from build123d import *

# Parameters (mm, degrees)
F0_W     = 50.8
F0_H     = 101.6
F1_DEPTH = 63.5
F2_R     = 12.7
F3_DEPTH = 96.52
F4_R     = 2.54
F5_DEPTH = 36.322
F6_R     = 6.35
F7_DEPTH = 12.7
F8_R     = 5.08


with BuildPart() as f1:
    # F0 (on Top) → F1 (new body)
    with BuildSketch(Plane.XY):
        Rectangle(F0_W, F0_H)
    extrude(amount=F1_DEPTH)

    # F2 (on face) → F3 (cut)
    with BuildSketch(Plane.XZ.offset(50.8)):
        with Locations((0, 25.4)):
            Circle(F2_R)
    extrude(amount=-F3_DEPTH, mode=Mode.SUBTRACT)

    # F4 (on face) → F5 (cut)
    with BuildSketch(Plane.XY.offset(63.5)):
        with Locations((0, 40.64)):
            Circle(F4_R)
    extrude(amount=-F5_DEPTH, mode=Mode.SUBTRACT)

    # F6 (on face) → F7 (cut)
    with BuildSketch(Plane.XY.offset(63.5)):
        Circle(F6_R)
    extrude(amount=-F7_DEPTH, mode=Mode.SUBTRACT)

    # F8
    f8_edges = [f1.edges().sort_by_distance(p)[0] for p in [
        (25.4, -50.8, 31.75),
        (-25.4, -50.8, 31.75),
        (-25.4, 50.8, 31.75),
        (-25.4, 0, 0),
        (0, 50.8, 0),
        (25.4, 50.8, 31.75),
        (25.4, 0, 0),
        (0, -50.8, 0),
    ]]
    fillet(f8_edges, radius=F8_R)


solid = f1.part
Model file for the job. Use its own axes, mm. A direction names the side the tool comes from. Round coordinates to 2 decimals unless told otherwise and drop trailing zeros. Order: outer loops, then holes, each group sorted by start corner. A loop starts at its lowest first (then second) coordinate and runs counter-clockwise, first axis right, second up.
(1) Band-saw the part on A-A (x = 0). List the corners of the cut face in (y, z).
(2) Drill centre lines: line 1 (X direction, y = 40.64, z = 48.25); line 2 (Y direction, x = 0, z = 49); line 3 (Z direction, x = 0, y = -18). Where is each one in solid material? Low to high.
(3) Pin check, flat tip, straight feed: pin 1 (7.5 mm diameter, centred on x = -2.5, z = 22, fed in from -Y). Stop position of the tip, or through.
(4) 3-axis set-ups, long thin cutter, end or side, ignore diameter. For faces 1 (the face through (5.86, -3.216, 14.133)), 2 (the face through (1.37, 42.78, 50.85)), 3 (the face through (23.872, 0.64, 1.449)): which of +Z, -Z, +X, -X, +Y, -Y reach the whole face in a straight line?
(5) Band-saw the part on B-B (y = 0). List the corners of the cut face in (x, z), then the cut area to 3 significant figures.
(6) Band-saw the part on C-C (z = 25.4). List the corners of the cut face in (x, y).
(7) Pull direction X, two halves, no side cores. Call faces 4 (the face through (-1.38, -6.2, 57.24)), 5 (the face through (0, 50.8, 34)), 6 (the face through (23.872, 49.351, 34.699)): released by +X, released by -X, zero draft, split by the parting line, or undercut.
(8) Band-saw the part on D-D (y = 40.64). List the corners of the cut face in (x, z), then the cut area to 3 significant figures.
Verdict:
1. outline: (-50.8, 5.08) arc R5.08 ccw to (-45.72, 0) - (45.72, 0) arc R5.08 ccw to (50.8, 5.08) - (50.8, 63.5) - (43.18, 63.5) - (43.18, 38.1) - (45.72, 38.1) - (45.72, 12.7) - (-50.8, 12.7) - close; (-50.8, 38.1) - (38.1, 38.1) - (38.1, 63.5) - (6.35, 63.5) - (6.35, 50.8) - (-6.35, 50.8) - (-6.35, 63.5) - (-50.8, 63.5) - close
2. line 1: x = -25.4 to -2.54, 2.54 to 25.4
2. line 2: y = -50.8 to 38.1, 43.18 to 50.8
2. line 3: z = 0 to 12.7, 38.1 to 63.5
3. pin 1: stops at y = 45.72
4. face 1: -Y
4. face 2: +Z
4. face 3: -Z, +X, +Y, -Y
5. outline: (-25.4, 5.08) arc R5.08 ccw to (-20.32, 0) - (20.32, 0) arc R5.08 ccw to (25.4, 5.08) - (25.4, 63.5) - (6.35, 63.5) - (6.35, 50.8) - (-6.35, 50.8) - (-6.35, 63.5) - (-25.4, 63.5) - close; hole circle Ø25.4 at (0, 25.4)
5. area: 2,550 mm2
6. outline: (-25.4, -45.72) arc R5.08 ccw to (-20.32, -50.8) - (-12.7, -50.8) - (-12.7, 45.72) - (12.7, 45.72) - (12.7, -50.8) - (20.32, -50.8) arc R5.08 ccw to (25.4, -45.72) - (25.4, 45.72) arc R5.08 ccw to (20.32, 50.8) - (-20.32, 50.8) arc R5.08 ccw to (-25.4, 45.72) - close
7. face 4: undercut
7. face 5: zero draft
7. face 6: released by +X
8. outline: (-25.4, 5.08) arc R5.08 ccw to (-20.32, 0) - (20.32, 0) arc R5.08 ccw to (25.4, 5.08) - (25.4, 63.5) - (2.54, 63.5) - (2.54, 37.84) arc R12.7 cw (long way) to (-2.54, 37.84) - (-2.54, 63.5) - (-25.4, 63.5) - close
8. area: 2,580 mm2
